Autodesk Inventor part; units mm, degrees
ref_plane "YZ Plane" through (0, 0, 0) normal (1, 0, 0) x (0, 1, 0)
ref_plane "XZ Plane" through (0, 0, 0) normal (0, 1, 0) x (-1, 0, 0)
ref_plane "XY Plane" through (0, 0, 0) normal (0, 0, 1) x (1, 0, 0)
sketch "Sketch1" plane through (0, 0, 0) normal (0, 1, 0) x (-1, 0, 0)
  arc A0 (2.5, 0) -> (-2.5, 0) centre (0, 0) ccw
  line L0 (2.5, 0) -> (2.5, -33)
  line L1 (-2.5, 0) -> (-2.5, -33)
  arc A1 (-2.5, -33) -> (2.5, -33) centre (0, -33) ccw
  circle A2 centre (0, -16.5) radius 2
  circle A3 centre (0, 0) radius 1.5
  circle A4 centre (0, -33) radius 1.5
  dimension "d11" = 5
  dimension "d12" = 33
  dimension "d13" = 33
  dimension "d14" = 5
  dimension "d15" = 4
  dimension "d16" = 3
  dimension "d17" = 3
extrude "Extrusion1" add sketch "Sketch1" along normal blind 2
properties part number "g_servo horn"
Design review of the part built by this model. Coordinates are the model's own, in mm. Give positions to 0.01 mm unless a question says otherwise; leave off trailing zeros. Write each loop counter-clockwise with the first axis right and the second up, starting at its lowest first coordinate (ties: lowest second). Pieces come first, ordered by that corner, then holes. Notation, with made-up numbers: M 65.25,-35 L 81.25,-35 A22 cw 81.25,-28 Z; hole C 26,17 d8. An arc over 180 degrees is marked long. Return JSON: item names as keys, results as strings. Group by question number.
Item 1: Take a section at C-C (y = 1). Give the boundary of the cut face in (x, z), plus the area to 3 significant figures.
Item 2: Take a section at A-A (x = 0). Give the boundary of the cut face in (y, z).
Item 3: The part is to be moulded in two halves that separate along Z. For faces 1 (the flat face through (-2.2, 2, -16.2)), 2 (the cylindrical face through (-0.1, 1, -35.5)), 3 (the cylindrical face through (0.325, 0.986, -31.536)), say which applies: pulls with the +Z half, pulls with the -Z half, needs draft (parallel to the pull), parting line crosses it, or undercut.
Item 4: Wall thickness on line 1 along Z through (x, y) = (0.1, 0.5); line 2 along Z through (x, y) = (-0.55, 0.9); line 3 along X through (y, z) = (0.35, -17): over which ranges is each line inside the solid? List them lowest first.
Item 5: Take a section at B-B (z = -16.5). Give the boundary of the cut face in (x, y), plus the area to 3 significant figures.
Return value:
{
 "1": {"outline": "M -2.5,-33 A2.5 ccw 2.5,-33 L 2.5,0 A2.5 ccw -2.5,0 Z; hole C 0,-16.5 d4; hole C 0,-33 d3; hole C 0,0 d3", "area": "158 mm2"},
 "2": {"outline": "M 0,-35.5 L 2,-35.5 L 2,-34.5 L 0,-34.5 Z; M 0,-31.5 L 2,-31.5 L 2,-18.5 L 0,-18.5 Z; M 0,-14.5 L 2,-14.5 L 2,-1.5 L 0,-1.5 Z; M 0,1.5 L 2,1.5 L 2,2.5 L 0,2.5 Z"},
 "3": {"face 1": "needs draft", "face 2": "pulls with the -Z half", "face 3": "undercut"},
 "4": {"line 1": "z = -35.5 to -34.5, -31.5 to -18.5, -14.5 to -1.5, 1.5 to 2.5", "line 2": "z = -35.44 to -34.4, -31.6 to -18.42, -14.58 to -1.4, 1.4 to 2.44", "line 3": "x = -2.5 to -1.94, 1.94 to 2.5"},
 "5": {"outline": "M -2.5,0 L -2,0 L -2,2 L -2.5,2 Z; M 2,0 L 2.5,0 L 2.5,2 L 2,2 Z", "area": "2.00 mm2"}
}
